Geometry check sheet. Reference: the model listing, model coordinates, mm. Face numbers are marked on the shaded views. A direction names the side the tool comes from. Give positions to 0.01 mm unless a question says otherwise; leave off trailing zeros. Loops run counter-clockwise (first coordinate to the right, second up) from the corner with the lowest first, then second, coordinate; pieces in that order, holes last. Notation, with made-up numbers: (81, -4.5) -> (98, -4.5) arc R22 cw to (98, 21.5) -> close; hole circle Ø3 at (-2, 74). An arc over 180 degrees is marked (long way). One line per question, with ' | ' between items.
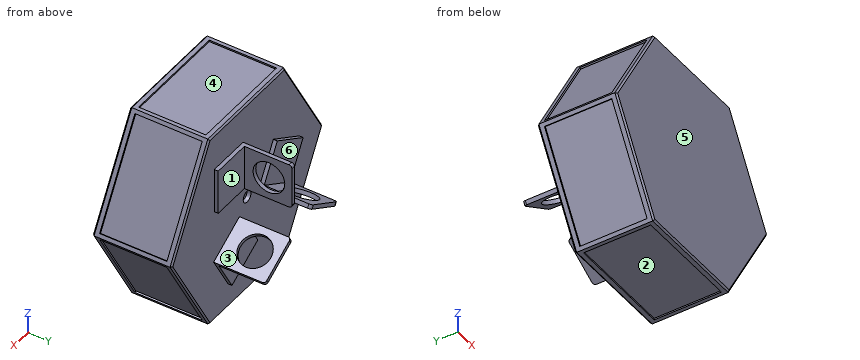
from build123d import *

# Parameters (mm, degrees)
BOSS_EXTRUDE1_DEPTH      = 100
SKETCH2_W                = 5
SKETCH2_H                = 57
BOSS_EXTRUDE2_DEPTH      = 65
SKETCH3_R                = 20
CUT_EXTRUDE1_DEPTH       = 257.915041827
SKETCH7_W                = 57
SKETCH7_H                = 5
BOSS_EXTRUDE3_DEPTH      = 50
FILLET1_R                = 3.6
SKETCH6_W                = 135
SKETCH6_H                = 85
CUT_EXTRUDE2_DEPTH       = 2
CIRPATTERN1_COUNT        = 3
FILLET1_OF_CIRPATTERN1_R = 3.6
CIRPATTERN2_COUNT        = 6
CHAMFER1_SIZE            = 2
SKETCH8_R                = 7.5
CUT_EXTRUDE3_DEPTH       = 5


with BuildPart() as part:
    # Sketch1 → Boss-Extrude1 (new body)
    with BuildSketch(Plane(origin=(0, 0, 0), x_dir=(1, 0, 0), z_dir=(0, 1, 0))):
        Polygon((72.168783649, 125), (-72.168783649, 125), (-144.337567297, 0), (-72.168783649, -125), (72.168783649, -125), (144.337567297, 0), align=None)
    extrude(amount=BOSS_EXTRUDE1_DEPTH)

    # Sketch2 → Boss-Extrude2 (add)
    with BuildSketch(Plane(origin=(0, 100, 0), x_dir=(1, 0, 0), z_dir=(0, 1, 0))):
        with Locations((10.331216351, -50)):
            Rectangle(SKETCH2_W, SKETCH2_H)
    boss_extrude2 = extrude(amount=BOSS_EXTRUDE2_DEPTH)

    # Sketch3 → Cut-Extrude1 (cut, through all)
    with BuildSketch(Plane.ZY.offset(-7.831216351)):
        with Locations((50, 136)):
            Circle(SKETCH3_R)
    cut_extrude1 = extrude(amount=-CUT_EXTRUDE1_DEPTH, mode=Mode.SUBTRACT)

    # Sketch7 → Boss-Extrude3 (add)
    with BuildSketch(Plane(origin=(12.831216351, 0, 0), x_dir=(0, 0, -1), z_dir=(1, 0, 0))):
        with Locations((-50, 102.5)):
            Rectangle(SKETCH7_W, SKETCH7_H)
    boss_extrude3 = extrude(amount=BOSS_EXTRUDE3_DEPTH)

    # Fillet1
    fillet1_edges = [part.edges().sort_by_distance(p)[0] for p in [
        (10.331216351, 165, 78.5),
        (10.331216351, 165, 21.5),
    ]]
    fillet(fillet1_edges, radius=FILLET1_R)

    # Sketch6 → Cut-Extrude2 (cut)
    with BuildSketch(Plane.XY.offset(125)):
        with Locations((0, 50)):
            Rectangle(SKETCH6_W, SKETCH6_H)
    cut_extrude2 = extrude(amount=-CUT_EXTRUDE2_DEPTH, mode=Mode.SUBTRACT)

    # CirPattern1: Boss-Extrude2, Cut-Extrude1, Boss-Extrude3 ×3 about axis
    cirpattern1_axis = Axis((0, 0, 0), (0, 1, 0))
    add([boss_extrude2.rotate(cirpattern1_axis, i * 360 / CIRPATTERN1_COUNT) for i in range(1, CIRPATTERN1_COUNT)])
    add([cut_extrude1.rotate(cirpattern1_axis, i * 360 / CIRPATTERN1_COUNT) for i in range(1, CIRPATTERN1_COUNT)], mode=Mode.SUBTRACT)
    add([boss_extrude3.rotate(cirpattern1_axis, i * 360 / CIRPATTERN1_COUNT) for i in range(1, CIRPATTERN1_COUNT)])

    # Fillet1 of CirPattern1
    fillet1_of_cirpattern1_edges = [part.edges().sort_by_distance(p)[0] for p in [
        (62.817386021, 165, -48.197095812),
        (13.453938006, 165, -19.697095812),
        (-73.148602373, 165, -30.302904188),
        (-23.785154357, 165, -1.802904188),
    ]]
    fillet(fillet1_of_cirpattern1_edges, radius=FILLET1_OF_CIRPATTERN1_R)

    # CirPattern2: Cut-Extrude2 ×6 about axis
    cirpattern2_axis = Axis((0, 0, 0), (0, 1, 0))
    for i in range(1, CIRPATTERN2_COUNT):
        add(cut_extrude2.rotate(cirpattern2_axis, i * 360 / CIRPATTERN2_COUNT), mode=Mode.SUBTRACT)

    # Chamfer1
    chamfer1_edges = [part.edges().sort_by_distance(p)[0] for p in [
        (-108.253175473, 100, -62.5),
        (-108.253175473, 100, 62.5),
        (0, 100, 125),
        (108.253175473, 100, 62.5),
        (108.253175473, 100, -62.5),
        (108.253175473, 0, 62.5),
        (0, 0, 125),
        (-108.253175473, 0, 62.5),
        (0, 100, -125),
        (-108.253175473, 0, -62.5),
        (0, 0, -125),
        (108.253175473, 0, -62.5),
    ]]
    chamfer(chamfer1_edges, length=CHAMFER1_SIZE)

    # Sketch8 → Cut-Extrude3 (cut)
    with BuildSketch(Plane(origin=(0, 100, 0), x_dir=(1, 0, 0), z_dir=(0, 1, 0))):
        with Locations(Location((0, 0, 0), (0, 0, 270))):
            Circle(SKETCH8_R)
    extrude(amount=-CUT_EXTRUDE3_DEPTH, mode=Mode.SUBTRACT)


solid = part.part
Item 1: Sectioned sample at D-D (x = 92). Record the cut outline in (y, z).
Result:
outline: (0, -86.65) -> (2, -90.65) -> (7.5, -90.65) -> (7.5, -86.65) -> (92.5, -86.65) -> (92.5, -90.65) -> (98, -90.65) -> (100, -86.65) -> (100, 86.65) -> (98, 90.65) -> (92.5, 90.65) -> (92.5, 86.65) -> (7.5, 86.65) -> (7.5, 90.65) -> (2, 90.65) -> (0, 86.65) -> close
Item 2: Depth check by flat-ended pin: pin 1 Ø6 at (x, y) = (-23.5, 16.5) entering from +Z; pin 2 Ø1.5 at (x, y) = (34.5, 82.5) entering from -Z; pin 3 Ø1 at (x, z) = (-33.5, -124) entering from +Y. Enter the tip coordinate at first touch or a pass-through.
Result:
pin 1: z = 123 | pin 2: z = -123 | pin 3: y = 99.5
Item 3: Release check for a two-part mould opening along X. For the marked faces 1, 2, 3 and 4 record: pulls with the +X half, pulls with the -X half, needs draft (parallel to the pull), parting line crosses it, or undercut.
Result:
face 1: needs draft | face 2: undercut | face 3: pulls with the +X half | face 4: undercut
Item 4: Set-up check for the marked faces 5 and 6: record each of +Z, -Z, +X, -X, +Y, -Y from which the full face is reachable in a straight line by a thin tool's end or side.
Result:
face 5: +Z, -Z, +X, -X, -Y | face 6: +Z, -X, +Y
Item 5: Sectioned sample at A-A (y = 108.5). Record the cut outline in (x, z).
Result:
outline: (-74.4, -28.14) -> (-71.9, -32.47) -> (-22.54, -3.97) -> (-25.04, 0.36) -> close; (7.83, 21.5) -> (12.83, 21.5) -> (12.83, 78.5) -> (7.83, 78.5) -> close; (12.2, -21.86) -> (61.57, -50.36) -> (64.07, -46.03) -> (14.7, -17.53) -> close
Item 6: Scan lines: probe 1 along Y at (x, z) = (-107.5, 9); probe 2 along Z at (x, y) = (-33, 10); probe 3 along Y at (x, z) = (39, -80). Record each from-to range of solid material in increasing order.
Result:
probe 1: 0 to 100 | probe 2: -123 to 123 | probe 3: 0 to 105
Item 7: Sectioned sample at B-B (z = 50). Record the cut outline in (x, y), plus the area to 3 significant figures.
Result:
outline: (-115.47, 2) -> (-113.16, 0) -> (113.16, 0) -> (115.47, 2) -> (115.47, 7.5) -> (113.16, 7.5) -> (113.16, 92.5) -> (115.47, 92.5) -> (115.47, 98) -> (113.16, 100) -> (62.83, 100) -> (62.83, 105) -> (12.83, 105) -> (12.83, 116) -> (7.83, 116) -> (7.83, 100) -> (-113.16, 100) -> (-115.47, 98) -> (-115.47, 92.5) -> (-113.16, 92.5) -> (-113.16, 7.5) -> (-115.47, 7.5) -> close; (7.83, 156) -> (12.83, 156) -> (12.83, 165) -> (7.83, 165) -> close | area: 23,100 mm2
